Here's the drawing with two shaded views (mm, measured from the low corner). I have some questions. A direction names the side the tool comes from. Coordinates: 2 decimals unless noted, no trailing zeros. Write each loop counter-clockwise with the first axis right and the second up, starting at its lowest first coordinate (ties: lowest second). Pieces come first, ordered by that corner, then holes.
Item 1: If we section it at C-C (y = 12): Please give me the cut outline in (x, z).
Item 2: If we section it at B-B (z = 7.75): Please give me the cut outline in (x, y).
Item 3: If I drill on line 1 (X direction, y = 3, z = 6.5); line 2 (Y direction, x = 21, z = 7.6); line 3 (X direction, y = 17, z = 1), over which ranges is the centre line in solid material (lowest first)?
Item 4: We'd pull the mould along X, two halves only. Please class the marked faces 1, 2 and 3: +X half, -X half, draft (parallel to the pull), parting line (faces both ways), or undercut.
Item 5: If we section it at A-A (z = 1): Please give me the cut outline in (x, y).
Item 6: If we section it at D-D (x = 14.5): Please give me the cut outline in (y, z).
Item 7: For the marked faces 4 and 5, which set-ups out of +Z, -Z, +X, -X, +Y, -Y let a thin tool reach every point of the face, with its end or its side?
Item 8: I'm going to push flat-ended pins straight in: pin 1 Ø2 at (x, y) = (21, 3) entering from +Z; pin 2 Ø3 at (x, y) = (12, 16.5) entering from -Z. Where does each tip first touch, or does it pass through?
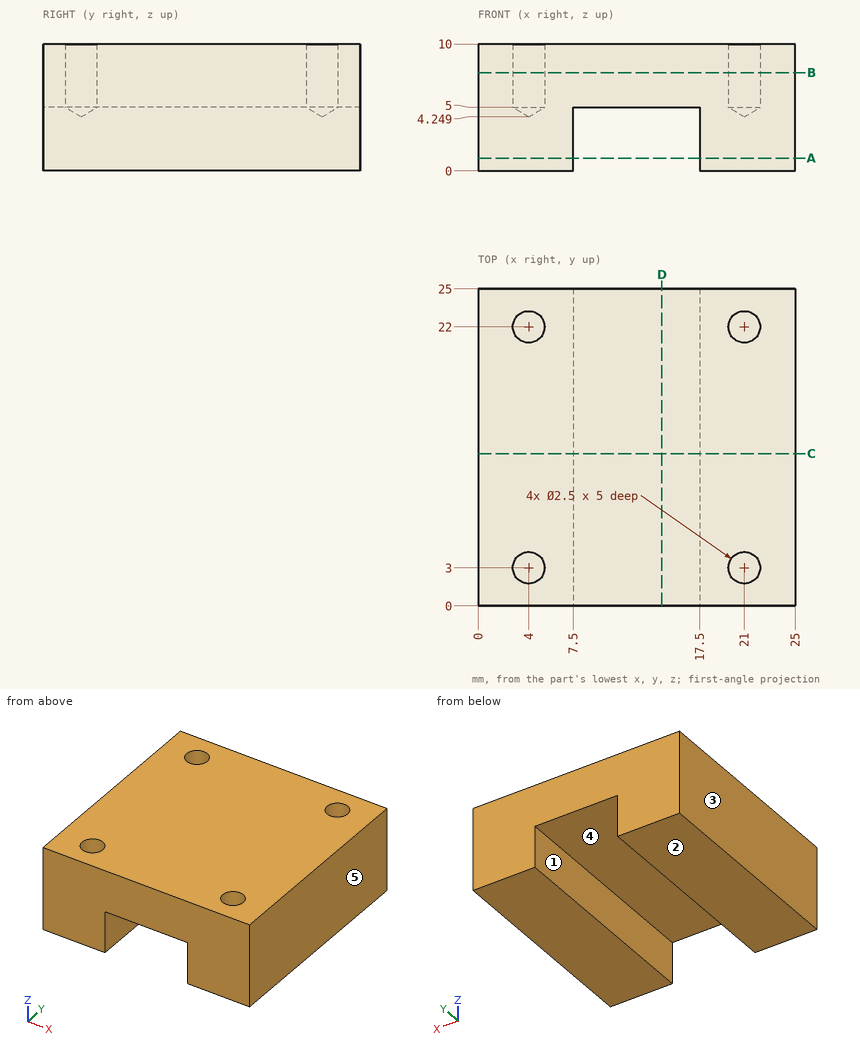
Answer list:
1. outline: (0, 0) - (7.5, 0) - (7.5, 5) - (17.5, 5) - (17.5, 0) - (25, 0) - (25, 10) - (0, 10) - close
2. outline: (0, 0) - (25, 0) - (25, 25) - (0, 25) - close; hole circle Ø2.5 at (4, 3); hole circle Ø2.5 at (4, 22); hole circle Ø2.5 at (21, 3); hole circle Ø2.5 at (21, 22)
3. line 1: x = 0 to 2.75, 5.25 to 19.75, 22.25 to 25
3. line 2: y = 0 to 1.75, 4.25 to 20.75, 23.25 to 25
3. line 3: x = 0 to 7.5, 17.5 to 25
4. face 1: undercut
4. face 2: draft
4. face 3: -X half
5. outline: (0, 0) - (7.5, 0) - (7.5, 25) - (0, 25) - close; (17.5, 0) - (25, 0) - (25, 25) - (17.5, 25) - close
6. outline: (0, 5) - (25, 5) - (25, 10) - (0, 10) - close
7. face 4: -Z, +Y, -Y
7. face 5: +Z, -Z, +X, +Y, -Y
8. pin 1: stops at z = 4.85
8. pin 2: stops at z = 5
